Design review of the part built by this model. Coordinates are the model's own, in mm. Give positions to 0.01 mm unless a question says otherwise; leave off trailing zeros. Write each loop counter-clockwise with the first axis right and the second up, starting at its lowest first coordinate (ties: lowest second). Pieces come first, ordered by that corner, then holes. Notation, with made-up numbers: (20, 40) - (77, 40) arc R19 ccw to (77, 54) - close; hole circle Ø11 at (14.25, -10). An arc over 180 degrees is marked (long way). Use a Markdown table: item, result. Add a question column.
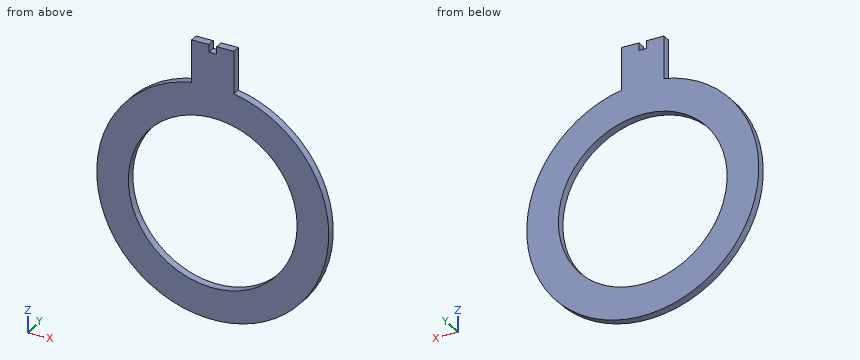
```python
from build123d import *

# Parameters (mm, degrees)
SKETCH1_R           = 50.8
BOSS_EXTRUDE1_DEPTH = 4.7625


with BuildPart() as part:
    # Sketch1 → Boss-Extrude1 (new body)
    with BuildSketch(Plane(origin=(0, 0, 0), x_dir=(1, 0, 0), z_dir=(0, 1, 0))):
        with BuildLine():
            Line((12.7, -94.085751798), (12.7, -68.685751798))
            ThreePointArc((12.7, -68.685751798), (0, 69.85), (-12.7, -68.685751798))
            Line((-12.7, -68.685751798), (-12.7, -94.085751798))
            Line((-12.7, -94.085751798), (-2.38125, -94.085751798))
            Line((-2.38125, -94.085751798), (-2.38125, -89.521371798))
            Line((-2.38125, -89.521371798), (2.38125, -89.521371798))
            Line((2.38125, -89.521371798), (2.38125, -94.085751798))
            Line((2.38125, -94.085751798), (12.7, -94.085751798))
        make_face()
        Circle(SKETCH1_R, mode=Mode.SUBTRACT)
    extrude(amount=BOSS_EXTRUDE1_DEPTH)


solid = part.part
```
(1) Add section A-A (x = 0). State the section outline as (y, z) points, and give its area (3 significant figures).
(2) Add section C-C (y = 4). State the section outline as (x, z) points, and give its area (3 significant figures).
(3) For line 1 along X through (y, z) = (2.6, 0); line 2 along Z through (x, y) = (-11.5, 4.55); line 3 along Z through (x, y) = (-38, 2.05), list the stretches that pass through material, from the lowest coordinate up.
(4) Add section D-D (z = -54). State the section outline as (x, y) points, and give its area (3 significant figures).
(5) Add section B-B (z = 0). State the section outline as (x, y) points, and give its area (3 significant figures).
(6) Insertion check: pin 1 (1.4 mm diameter, centred on y = 2, z = 91.5, fed in from -X); pin 2 (1.4 mm diameter, centred on y = 3, z = 91.5, fed in from +X); pin 3 (8 mm diameter, centred on x = -49, z = -10, fed in from -Y); pin 4 (2.5 mm diameter, centred on x = 0, y = 3.5, fed in from +Z). Each pin has a flat end and moves straight along its axis. Give the tip position at first contact, or say it passes through.
Answers follow:
| question | item | result |
|---|---|---|
| 1 | outline | (0, -69.85) - (4.76, -69.85) - (4.76, -50.8) - (0, -50.8) - close; (0, 50.8) - (4.76, 50.8) - (4.76, 89.52) - (0, 89.52) - close |
| 1 | area | 275 mm^2 |
| 2 | outline | (-12.7, 68.69) arc R69.85 ccw (long way) to (12.7, 68.69) - (12.7, 94.09) - (2.38, 94.09) - (2.38, 89.52) - (-2.38, 89.52) - (-2.38, 94.09) - (-12.7, 94.09) - close; hole circle Ø101.6 at (0, 0) |
| 2 | area | 7,820 mm^2 |
| 3 | line 1 | -69.85 to -50.8, 50.8 to 69.85 |
| 3 | line 2 | -68.9 to -49.48, 49.48 to 94.09 |
| 3 | line 3 | -58.61 to -33.71, 33.71 to 58.61 |
| 4 | outline | (-44.31, 0) - (44.31, 0) - (44.31, 4.76) - (-44.31, 4.76) - close |
| 4 | area | 422 mm^2 |
| 5 | outline | (-69.85, 0) - (-50.8, 0) - (-50.8, 4.76) - (-69.85, 4.76) - close; (50.8, 0) - (69.85, 0) - (69.85, 4.76) - (50.8, 4.76) - close |
| 5 | area | 181 mm^2 |
| 6 | pin 1 | x = -12.7 |
| 6 | pin 2 | x = 12.7 |
| 6 | pin 3 | y = 0 |
| 6 | pin 4 | z = 89.52 |
